The model under review builds one solid part; all positions refer to its coordinate system, in mm. Coordinates: 2 decimals unless noted, no trailing zeros. Loops run counter-clockwise (first coordinate to the right, second up) from the corner with the lowest first, then second, coordinate; pieces in that order, holes last. Notation, with made-up numbers: (67, 77) - (106, 77) arc R28 ccw to (106, 108) - close; hole circle Ø2 at (68, 74.5). An arc over 180 degrees is marked (long way). Answer in a Markdown table with one row per item. Add a question column.
(1) We need section A-A on z = 26.5. Write out the cut boundary in (x, y).
(2) For P1, Ø5, axis at x = -6.5, y = 3.5, coming from the -Z side; P2, Ø3.5, axis at y = 16, z = 11, coming from the -X side; P3, Ø14.5, axis at x = -2.5, y = 18, coming from the +Z side, all flat-tipped, find the tip position at first contact; note any pin that passes through.
(3) We need section C-C on x = 0. Write out the cut boundary in (y, z), plus the area to 3 significant figures.
(4) For line 1 along X through (y, z) = (20, 5); line 2 along Y through (x, z) = (9.35, 11); line 3 along Z through (x, y) = (0, 21), list the stretches that pass through material, from the lowest coordinate up.
(5) We need section B-B on y = 7. Write out the cut boundary in (x, z).
(6) We need section D-D on z = 5.5. Write out the cut boundary in (x, y), plus the area to 3 significant figures.
from build123d import *

# Parameters (mm, degrees)
F2_DEPTH      = 6
F3_R          = 21
F4_DEPTH      = 102.501
F4_DEPTH_BACK = 102.501
F5_DEPTH      = 28
F5_DEPTH_BACK = 5
F6_R          = 10.25
F7_DEPTH      = 30.3
F9_D          = 3


with BuildPart() as f2:
    # F1 (on Front) → F2 (new body)
    with BuildSketch(Plane.XZ):
        with BuildLine():
            ThreePointArc((6.5, -102.5), (10.7426406871, -100.7426406871), (12.5, -96.5))
            Line((12.5, -96.5), (12.5, 96.5))
            ThreePointArc((12.5, 96.5), (10.7426406871, 100.7426406871), (6.5, 102.5))
            Line((6.5, 102.5), (-6.5, 102.5))
            ThreePointArc((-6.5, 102.5), (-10.7426406871, 100.7426406871), (-12.5, 96.5))
            Line((-12.5, 96.5), (-12.5, -96.5))
            ThreePointArc((-12.5, -96.5), (-10.7426406871, -100.7426406871), (-6.5, -102.5))
            Line((-6.5, -102.5), (6.5, -102.5))
        make_face()
    extrude(amount=F2_DEPTH)

    # F3 (on Top) → F4 (cut, two sides)
    with BuildSketch(Plane.XY) as f4_sk:
        with Locations((0, 16)):
            Circle(F3_R)
    extrude(amount=-F4_DEPTH, mode=Mode.SUBTRACT)
    extrude(f4_sk.sketch, amount=F4_DEPTH_BACK, mode=Mode.SUBTRACT)

    # F0 (on Front) → F5 (join, two sides)
    with BuildSketch(Plane.XZ) as f5_sk:
        with BuildLine():
            Line((-6.5, -100.5), (6.5, -100.5))
            ThreePointArc((6.5, -100.5), (9.3284271247, -99.3284271247), (10.5, -96.5))
            Line((10.5, -96.5), (10.5, 96.5))
            ThreePointArc((10.5, 96.5), (9.3284271247, 99.3284271247), (6.5, 100.5))
            Line((6.5, 100.5), (-6.5, 100.5))
            ThreePointArc((-6.5, 100.5), (-9.3284271247, 99.3284271247), (-10.5, 96.5))
            Line((-10.5, 96.5), (-10.5, -96.5))
            ThreePointArc((-10.5, -96.5), (-9.3284271247, -99.3284271247), (-6.5, -100.5))
        make_face()
    extrude(amount=-F5_DEPTH)
    extrude(f5_sk.sketch, amount=F5_DEPTH_BACK)

    # F6 (on face) → F7 (cut)
    with BuildSketch(Plane(origin=(0, 28, 0), x_dir=(-1, 0, 0), z_dir=(0, 1, 0))):
        with Locations((0, 5.5)):
            Circle(F6_R)
    extrude(amount=-F7_DEPTH, mode=Mode.SUBTRACT)

    # F9 (through all)
    with Locations(Plane(origin=(-10.5, 0, 0), x_dir=(0, -1, 0), z_dir=(-1, 0, 0))):
        with Locations((-16, 11)):
            Hole(F9_D / 2)


solid = f2.part
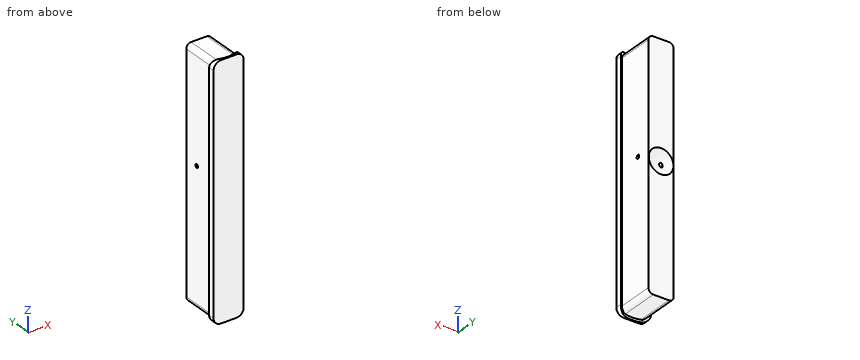
Outcome:
| question | item | result |
|---|---|---|
| 1 | outline | (-12.5, -6) - (12.5, -6) - (12.5, -0.87) arc R21 cw to (10.5, -2.19) - (10.5, 28) - (-10.5, 28) - (-10.5, -2.19) arc R21 cw to (-12.5, -0.87) - close |
| 2 | P1 | z = -100.5 |
| 2 | P2 | x = -10.5 |
| 2 | P3 | z = 100.5 |
| 3 | outline | (-6, -102.5) - (-5, -102.5) - (-5, -100.5) - (28, -100.5) - (28, -4.75) - (-2.3, -4.75) - (-2.3, 15.75) - (28, 15.75) - (28, 100.5) - (-5, 100.5) - (-5, 102.5) - (-6, 102.5) - close |
| 3 | area | 6,220 mm² |
| 4 | line 1 | -10.5 to -10.24, 10.24 to 10.5 |
| 4 | line 2 | -6 to 14.5, 17.5 to 28 |
| 4 | line 3 | -100.5 to -4.75, 15.75 to 100.5 |
| 5 | outline | (-10.5, -96.5) arc R4 ccw to (-6.5, -100.5) - (6.5, -100.5) arc R4 ccw to (10.5, -96.5) - (10.5, 96.5) arc R4 ccw to (6.5, 100.5) - (-6.5, 100.5) arc R4 ccw to (-10.5, 96.5) - close; hole circle Ø20.5 at (0, 5.5) |
| 6 | outline | (-12.5, -6) - (12.5, -6) - (12.5, -0.87) arc R21 cw to (10.5, -2.19) - (10.5, 28) - (10.25, 28) - (10.25, -2.3) - (-10.25, -2.3) - (-10.25, 28) - (-10.5, 28) - (-10.5, -2.19) arc R21 cw to (-12.5, -0.87) - close |
| 6 | area | 111 mm² |
